Source: CAD feature listing. Evaluate the final solid. Frame: model axes, mm. A direction names the side the tool comes from. Round coordinates to 2 decimals unless told otherwise and drop trailing zeros. Write each loop counter-clockwise with the first axis right and the second up, starting at its lowest first coordinate (ties: lowest second). Pieces come first, ordered by that corner, then holes. Notation, with made-up numbers: M 68,48 L 105,48 A32 cw 105,81 Z; hole C 59,40 d5. An arc over 180 degrees is marked long. Answer in a Markdown table with one row per item.
from build123d import *

# Parameters (mm, degrees)
F0_W     = 14
F0_H     = 14
F1_DEPTH = 2.3
F2_W     = 1.5
F2_H     = 2
F3_DEPTH = 11.7
F4_SIZE  = 0.4
F5_R     = 0.74999


# Not quite as in the source:
# - a fillet or chamfer is up to 0.001 mm smaller than in the source, because OpenCascade refuses the exact size


with BuildPart() as f1:
    # F0 (on Top) → F1 (new body)
    with BuildSketch(Plane.XY):
        with Locations((7, 7)):
            Rectangle(F0_W, F0_H)
    extrude(amount=F1_DEPTH)

    # F2 (on face) → F3 (join)
    with BuildSketch(Plane.XY.offset(2.3)):
        with Locations((0.75, 13)):
            Rectangle(F2_W, F2_H)
        with Locations((0.75, 1)):
            Rectangle(F2_W, F2_H)
        with Locations((13.25, 13)):
            Rectangle(F2_W, F2_H)
        with Locations((13.25, 1)):
            Rectangle(F2_W, F2_H)
        with Locations((0.75, 9)):
            Rectangle(F2_W, F2_H)
        with Locations((0.75, 5)):
            Rectangle(F2_W, F2_H)
        with Locations((13.25, 9)):
            Rectangle(F2_W, F2_H)
        with Locations((13.25, 5)):
            Rectangle(F2_W, F2_H)
        with Locations((4.9166666667, 9)):
            Rectangle(F2_W, F2_H)
        with Locations((9.0833333333, 9)):
            Rectangle(F2_W, F2_H)
        with Locations((4.9166666667, 13)):
            Rectangle(F2_W, F2_H)
        with Locations((9.0833333333, 13)):
            Rectangle(F2_W, F2_H)
        with Locations((4.9166666667, 5)):
            Rectangle(F2_W, F2_H)
        with Locations((9.0833333333, 5)):
            Rectangle(F2_W, F2_H)
        with Locations((4.9166666667, 1)):
            Rectangle(F2_W, F2_H)
        with Locations((9.0833333333, 1)):
            Rectangle(F2_W, F2_H)
    extrude(amount=F3_DEPTH)

    # F4
    f4_edges = [f1.edges().sort_by_distance(p)[0] for p in [
        (7, 0, 0),
        (0, 7, 0),
        (14, 7, 0),
        (7, 14, 0),
    ]]
    chamfer(f4_edges, length=F4_SIZE)

    # F5 (radius 0.75 in the source; OpenCascade refuses exactly that, so slightly less here)
    f5_edges = [f1.edges().sort_by_distance(p)[0] for p in [
        (14, 13, 14),
        (12.5, 13, 14),
        (9.833333, 13, 14),
        (8.333333, 13, 14),
        (5.666667, 13, 14),
        (4.166667, 13, 14),
        (1.5, 13, 14),
        (0, 13, 14),
        (0, 9, 14),
        (1.5, 9, 14),
        (4.166667, 9, 14),
        (5.666667, 9, 14),
        (8.333333, 9, 14),
        (9.833333, 9, 14),
        (12.5, 9, 14),
        (14, 9, 14),
        (14, 5, 14),
        (12.5, 5, 14),
        (9.833333, 5, 14),
        (8.333333, 5, 14),
        (5.666667, 5, 14),
        (4.166667, 5, 14),
        (1.5, 5, 14),
        (0, 5, 14),
        (0, 1, 14),
        (1.5, 1, 14),
        (4.166667, 1, 14),
        (5.666667, 1, 14),
        (8.333333, 1, 14),
        (9.833333, 1, 14),
        (12.5, 1, 14),
        (14, 1, 14),
    ]]
    fillet(f5_edges, radius=F5_R)


solid = f1.part
Q1. Pull-direction query (X, two-part tool) for faces 1 (the flat face through (13, 2, 8)), 2 (the flat face through (1.5, 13, 8)), 3 (the flat face through (0, 5, 7)); classes: pulls with the +X half, pulls with the -X half, needs draft (parallel to the pull), parting line crosses it, or undercut.
Solutions:
| item | result |
|---|---|
| face 1 | needs draft |
| face 2 | undercut |
| face 3 | pulls with the -X half |
Q2. Access query for faces 4 (the flat face through (13, 12, 8)), 5 (the flat face through (9.833, 1, 8)), 6 (the flat face through (5, 14, 7)). Directions: +Z, -Z, +X, -X, +Y, -Y. A direction counts if a zero-diameter tool reaches every point of the face in a straight line with its end or side. Return the directions, or none.
Solutions:
| item | result |
|---|---|
| face 4 | +Z, +X, -X |
| face 5 | +Z, +Y, -Y |
| face 6 | +Z, -Z, +X, -X, +Y |
Q3. Material intervals for probe 1 along Y at (x, z) = (0.75, 13); probe 2 along X at (y, z) = (9.5, 4.25); probe 3 along Z at (x, y) = (5.75, 7.5), sorted ascending.
Solutions:
| item | result |
|---|---|
| probe 1 | y = 0 to 2, 4 to 6, 8 to 10, 12 to 14 |
| probe 2 | x = 0 to 1.5, 4.17 to 5.67, 8.33 to 9.83, 12.5 to 14 |
| probe 3 | z = 0 to 2.3 |
Q4. Section C-C (z = 2.75). State how many separate pieces and enclosed holes the cut face has, and give its area (3 significant figures).
Solutions:
| item | result |
|---|---|
| separate pieces | 16 |
| enclosed holes | 0 |
| area | 48.0 mm2 |
Q5. Section D-D (x = 8.75). Return loops of the section in (y, z).
Solutions:
| item | result |
|---|---|
| outline | M 0,0.4 L 0.4,0 L 13.6,0 L 14,0.4 L 14,13.92 L 12,13.92 L 12,2.3 L 10,2.3 L 10,13.92 L 8,13.92 L 8,2.3 L 6,2.3 L 6,13.92 L 4,13.92 L 4,2.3 L 2,2.3 L 2,13.92 L 0,13.92 Z |
Q6. Section B-B (x = 2.5). Return loops of the section in (y, z).
Solutions:
| item | result |
|---|---|
| outline | M 0,0.4 L 0.4,0 L 13.6,0 L 14,0.4 L 14,2.3 L 0,2.3 Z |
Q7. Contact query for a flat-ended pin moving along its axis: pin 1 Ø8 at (x, y) = (7.5, 9) entering from +Z. Output: stop coordinate, or through.
Solutions:
| item | result |
|---|---|
| pin 1 | stops at z = 14 |
